Build history of the part. All positions in model axes, mm. A direction names the side the tool comes from. Give positions to 0.01 mm unless a question says otherwise; leave off trailing zeros. Write each loop counter-clockwise with the first axis right and the second up, starting at its lowest first coordinate (ties: lowest second). Pieces come first, ordered by that corner, then holes. Notation, with made-up numbers: (-5.75, 6) -> (20.25, 6) arc R24 cw to (20.25, 35) -> close; hole circle Ø1 at (30.5, 18). An arc over 180 degrees is marked (long way). Put each result on its own line as item: value. Start each with the question number.
Item 1: Slice it at C-C, the plane x = -40.5. List the corners of the cut face in (y, z).
Item 2: Slice it at D-D, the plane y = 9.5. List the corners of the cut face in (x, z).
Item 3: Slice it at B-B, the plane z = 1.5. List the corners of the cut face in (x, y).
Item 4: Drill centre lines: line 1 along X through (y, z) = (27, 4); line 2 along Z through (x, y) = (-19.5, 48); line 3 along Y through (x, z) = (28, 22.5). Where is each one in solid material? Low to high.
Item 5: Tool access for faces 5 (the flat face through (-14.22, 39.417, -0.098)), 6 (the flat face through (16.354, 7.387, -9.643)), 7 (the flat face through (63, 31, -33.5)): list every direction of +Z, -Z, +X, -X, +Y, -Y with a clear straight run to the whole face (end or side of a thin tool).
Item 6: Two-plate mould, pull along X, no slides. Class faces 1 (the cylindrical face through (-48.279, 13.604, -0.098)), 2 (the flat face through (26.65, 12.48, -17.76)), 3 (the cylindrical face through (-6.495, 13.449, -0.098)), 4 (the flat face through (20.69, 11.56, 24.52)): pulls with the +X half, pulls with the -X half, needs draft (parallel to the pull), parting line crosses it, or undercut.
Item 7: Flat gauge pins, fed straight in: pin 1 Ø6 at (y, z) = (11, -12) entering from +X; pin 2 Ø4 at (y, z) = (41.5, 14) entering from +X. Where does each tip first touch, or does it go through?
Item 8: Slice it at A-A, the plane y = 24.5. List the corners of the cut face in (x, z), plus the area to 3 significant figures.
```python
from build123d import *

# Parameters (mm, degrees)
Y_KSEKLIK_EKSTR_ZYON1_DEPTH = 55
KES_EKSTR_ZYON1_DEPTH       = 55
KES_EKSTR_ZYON1_DEPTH_BACK  = 55
IZIM4_R                     = 20.5
IZIM4_R_2                   = 6
KES_EKSTR_ZYON2_DEPTH       = 55
KES_EKSTR_ZYON2_DEPTH_BACK  = 55
KES_EKSTR_ZYON3_DEPTH       = 107.314994316
KES_EKSTR_ZYON3_DEPTH_BACK  = 107.314994316


with BuildPart() as part:
    # Çizim2 → Yükseklik-Ekstrüzyon1 (new body)
    with BuildSketch(Plane(origin=(0, 0, 0), x_dir=(1, 0, 0), z_dir=(0, 1, 0))):
        with BuildLine():
            Line((-60.70745329, -7), (-0.70745329, -7))
            ThreePointArc((-0.70745329, -7), (1.083042474, -7.331582183), (2.636059642, -8.282350033))
            Line((2.636059642, -8.282350033), (39.256799322, -41.217649967))
            ThreePointArc((39.256799322, -41.217649967), (40.809816489, -42.168417817), (42.600312254, -42.5))
            Line((42.600312254, -42.5), (80.446429482, -42.5))
            Line((80.446429482, -42.5), (80.446429482, -33.5))
            Line((80.446429482, -33.5), (45.577301243, -33.5))
            ThreePointArc((45.577301243, -33.5), (43.771367773, -33.162467619), (42.209258712, -32.19544172))
            Line((42.209258712, -32.19544172), (10.967785126, -3.72181941))
            ThreePointArc((10.967785126, -3.72181941), (9.335858983, -0.008678576), (10.994031787, 3.692815818))
            Line((10.994031787, 3.692815818), (42.741966981, 32.219193509))
            ThreePointArc((42.741966981, 32.219193509), (44.294345006, 33.168831093), (46.083762852, 33.5))
            Line((46.083762852, 33.5), (80.446429482, 33.5))
            Line((80.446429482, 33.5), (80.446429482, 42.5))
            Line((80.446429482, 42.5), (42.634342581, 42.5))
            ThreePointArc((42.634342581, 42.5), (40.844924735, 42.168831093), (39.29254671, 41.219193509))
            Line((39.29254671, 41.219193509), (2.634342581, 8.280806491))
            ThreePointArc((2.634342581, 8.280806491), (1.081964556, 7.331168907), (-0.70745329, 7))
            Line((-0.70745329, 7), (-60.70745329, 7))
            Line((-60.70745329, 7), (-60.70745329, -7))
        make_face()
    extrude(amount=Y_KSEKLIK_EKSTR_ZYON1_DEPTH)

    # Çizim4 → Kes-Ekstrüzyon1 (cut, two sides: drawn at the far end of the back side and taken through both)
    with BuildSketch(Plane.XY.offset(-KES_EKSTR_ZYON1_DEPTH_BACK)):
        with BuildLine():
            Line((-28.975635888, 54.672444157), (68.446429482, 39.5))
            ThreePointArc((68.446429482, 39.5), (76.931710856, 35.985281374), (80.446429482, 27.5))
            Line((80.446429482, 27.5), (80.446429482, 55))
            Line((80.446429482, 55), (-33.207453133, 55))
            ThreePointArc((-33.207453133, 55), (-31.085215516, 54.917988745), (-28.975635888, 54.672444157))
        make_face()
        with BuildLine():
            Line((80.446429482, 0), (80.446429482, 27.5))
            ThreePointArc((80.446429482, 27.5), (76.931710856, 19.014718626), (68.446429482, 15.5))
            Line((68.446429482, 15.5), (-28.975635888, 0.327555843))
            ThreePointArc((-28.975635888, 0.327555843), (-31.085215594, 0.082011249), (-33.20745329, 0))
            Line((-33.20745329, 0), (80.446429482, 0))
        make_face()
        with BuildLine():
            ThreePointArc((-60.70745329, 27.5), (-52.652889717, 46.945436538), (-33.207453133, 55))
            Line((-33.207453133, 55), (-60.70745329, 55))
            Line((-60.70745329, 55), (-60.70745329, 27.5))
        make_face()
        with BuildLine():
            ThreePointArc((-33.20745329, 0), (-52.652889773, 8.054563517), (-60.70745329, 27.5))
            Line((-60.70745329, 27.5), (-60.70745329, 0))
            Line((-60.70745329, 0), (-33.20745329, 0))
        make_face()
        with Locations(Location((-33.20745329, 27.5, 0), (0, 0, 180))):
            Circle(IZIM4_R)
        with Locations(Location((68.446429482, 27.5, 0), (0, 0, 180))):
            Circle(IZIM4_R_2)
    extrude(amount=KES_EKSTR_ZYON1_DEPTH + KES_EKSTR_ZYON1_DEPTH_BACK, mode=Mode.SUBTRACT)

    # Çizim7 → Kes-Ekstrüzyon2 (cut, two sides: drawn at the far end of the back side and taken through both)
    with BuildSketch(Plane.XY.offset(-KES_EKSTR_ZYON2_DEPTH_BACK)):
        with BuildLine():
            Line((-15.614003465, 38.022382014), (-12.78557634, 40.850809138))
            Line((-12.78557634, 40.850809138), (-19.856644152, 47.92187695))
            Line((-19.856644152, 47.92187695), (-22.685071277, 45.093449825))
            ThreePointArc((-22.685071277, 45.093449825), (-18.711764276, 41.995689014), (-15.614003465, 38.022382014))
        make_face()
    extrude(amount=KES_EKSTR_ZYON2_DEPTH + KES_EKSTR_ZYON2_DEPTH_BACK, mode=Mode.SUBTRACT)

    # Çizim8 → Kes-Ekstrüzyon3 (cut, two sides: drawn at the far end of the back side and taken through both)
    with BuildSketch(Plane.XY.offset(-KES_EKSTR_ZYON3_DEPTH_BACK)):
        with BuildLine():
            Line((-1.827361747, 11.63999197), (-1.784643175, 11.646644931))
            Line((-1.784643175, 11.646644931), (1.558869757, 12.16736129))
            Line((1.558869757, 12.16736129), (38.179609438, 17.870649613))
            Line((38.179609438, 17.870649613), (41.52312237, 18.391365973))
            Line((41.52312237, 18.391365973), (50.029447873, 19.716135143))
            ThreePointArc((50.029447873, 19.716135143), (56.694891282, 27.5), (50.029447873, 35.283864857))
            Line((50.029447873, 35.283864857), (41.52312237, 36.608634027))
            Line((41.52312237, 36.608634027), (38.179609438, 37.129350387))
            Line((38.179609438, 37.129350387), (1.558869757, 42.83263871))
            Line((1.558869757, 42.83263871), (-1.784643175, 43.353355069))
            Line((-1.784643175, 43.353355069), (-1.827361747, 43.36000803))
            ThreePointArc((-1.827361747, 43.36000803), (-6.448805477, 41.607340849), (-7.306116969, 36.73963077))
            ThreePointArc((-7.306116969, 36.73963077), (-5.70745329, 27.5), (-7.306116969, 18.26036923))
            ThreePointArc((-7.306116969, 18.26036923), (-6.448805477, 13.392659151), (-1.827361747, 11.63999197))
        make_face()
    extrude(amount=KES_EKSTR_ZYON3_DEPTH + KES_EKSTR_ZYON3_DEPTH_BACK, mode=Mode.SUBTRACT)


solid = part.part
```
Values follow:
1. outline: (0.98, -7) -> (8.34, -7) -> (8.34, 7) -> (0.98, 7) -> close; (46.66, -7) -> (54.02, -7) -> (54.02, 7) -> (46.66, 7) -> close
2. outline: (-54, -7) -> (-43.02, -7) -> (-43.02, 7) -> (-54, 7) -> close; (-23.4, -7) -> (-0.71, -7) arc R5 cw to (2.63, -8.28) -> (29.92, -32.8) -> (29.92, -20.7) -> (10.99, -3.69) arc R5 cw to (10.97, 3.72) -> (29.92, 21) -> (29.92, 32.82) -> (2.64, 8.28) arc R5 cw to (-0.71, 7) -> (-23.4, 7) -> close
3. outline: (-28.98, 0.33) -> (9.56, 6.33) -> (9.56, 13.41) -> (-1.83, 11.64) arc R5 cw to (-7.31, 18.26) arc R27.5 ccw to (-7.31, 36.74) arc R5 cw to (-1.83, 43.36) -> (9.56, 41.59) -> (9.56, 48.67) -> (-28.98, 54.67) arc R27.5 ccw (long way) to start; hole (-22.69, 45.09) arc R20.5 ccw (long way) to (-15.61, 38.02) -> (-12.79, 40.85) -> (-19.86, 47.92) -> close
4. line 1: -60.7 to -53.7, -12.71 to -5.71
4. line 2: -7 to 7
4. line 3: 9.2 to 16.29, 38.71 to 45.8
5. face 5: +Z, -Z
5. face 6: +Z, -Z, +X, -Y
5. face 7: +X, +Y, -Y
6. face 1: undercut
6. face 2: pulls with the +X half
6. face 3: undercut
6. face 4: pulls with the -X half
7. pin 1: x = 23.58
7. pin 2: x = 24.44
8. outline: (-60.54, -7) -> (-53.49, -7) -> (-53.49, 7) -> (-60.54, 7) -> close; (-12.93, -7) -> (-5.87, -7) -> (-5.87, 7) -> (-12.93, 7) -> close; (56.1, -42.5) -> (63.25, -42.5) -> (63.25, -33.5) -> (56.1, -33.5) -> close; (56.1, 33.5) -> (63.25, 33.5) -> (63.25, 42.5) -> (56.1, 42.5) -> close; (73.64, -42.5) -> (80.07, -42.5) -> (80.07, -33.5) -> (73.64, -33.5) -> close; (73.64, 33.5) -> (80.07, 33.5) -> (80.07, 42.5) -> (73.64, 42.5) -> close
8. area: 442 mm2
